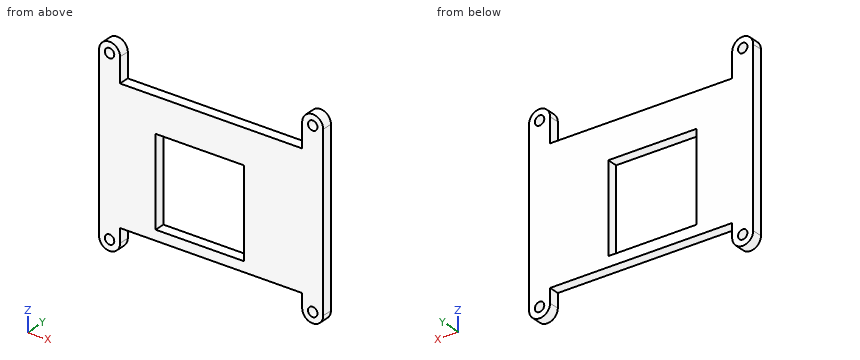
from build123d import *

# Parameters (mm, degrees)
SKETCH_1_R      = 1.35
SKETCH_1_W      = 25.2
SKETCH_1_H      = 25.2
EXTRUDE_1_DEPTH = 3


with BuildPart() as part:
    # 草图1 → 凸台-拉伸1 (new body)
    with BuildSketch(Plane(origin=(0, 0, 0), x_dir=(1, 0, 0), z_dir=(0, 1, 0))):
        with BuildLine():
            Line((-28.75, 19.5), (-28.75, -29.5))
            ThreePointArc((-28.75, -29.5), (-25.75, -32.5), (-22.75, -29.5))
            Line((-22.75, -29.5), (-22.75, -22.5))
            Line((-22.75, -22.5), (29.25, -22.5))
            Line((29.25, -22.5), (29.25, -29.5))
            ThreePointArc((29.25, -29.5), (32.25, -32.5), (35.25, -29.5))
            Line((35.25, -29.5), (35.25, 19.5))
            ThreePointArc((35.25, 19.5), (32.25, 22.5), (29.25, 19.5))
            Line((29.25, 19.5), (29.25, 15.5))
            Line((29.25, 15.5), (-22.75, 15.5))
            Line((-22.75, 15.5), (-22.75, 19.5))
            ThreePointArc((-22.75, 19.5), (-25.75, 22.5), (-28.75, 19.5))
        make_face()
        with Locations((-25.75, 19.5)):
            Circle(SKETCH_1_R, mode=Mode.SUBTRACT)
        with Locations((-25.75, -29.5)):
            Circle(SKETCH_1_R, mode=Mode.SUBTRACT)
        with Locations((32.25, 19.5)):
            Circle(SKETCH_1_R, mode=Mode.SUBTRACT)
        with Locations((32.25, -29.5)):
            Circle(SKETCH_1_R, mode=Mode.SUBTRACT)
        Rectangle(SKETCH_1_W, SKETCH_1_H, mode=Mode.SUBTRACT)
    extrude(amount=EXTRUDE_1_DEPTH)


solid = part.part
Could you check a few things on this model? Use its own coordinates, in mm. Give positions to 0.01 mm unless a question says otherwise; leave off trailing zeros. Write each loop counter-clockwise with the first axis right and the second up, starting at its lowest first coordinate (ties: lowest second). Pieces come first, ordered by that corner, then holes. Notation, with made-up numbers: (83, 28) -> (120, 28) arc R23 cw to (120, 55) -> close; hole circle Ø2 at (-39.5, 7.25). An arc over 180 degrees is marked (long way). Answer as CSV lines item,"result". Start each with the question number.
(1) If we section it at B-B, the plane x = 32.25: Write out the boundary of the cut face in (y, z), and give its area (3 significant figures).
(2) Please list where these lines run through material, in increasing order: line 1 (X direction, y = 1.45, z = 29.5); line 2 (Z direction, x = 32.25, y = 2.25).
(3) If we section it at A-A, the plane z = -3: Write out the boundary of the cut face in (x, y), and give its area (3 significant figures).
(4) If we section it at C-C, the plane y = 1.15: Write out the boundary of the cut face in (x, z).
(5) I'm going to push flat-ended pins straight in: pin 1 Ø1.5 at (x, y) = (-18.5, 1) entering from -Z; pin 2 Ø0.9 at (x, y) = (2, 2) entering from +Z. Where does each tip first touch, or does it pass through?
(6) If we section it at D-D, the plane x = 10: Write out the boundary of the cut face in (y, z), and give its area (3 significant figures).
Answer list:
1,outline,"(0, -22.5) -> (3, -22.5) -> (3, -20.85) -> (0, -20.85) -> close; (0, -18.15) -> (3, -18.15) -> (3, 28.15) -> (0, 28.15) -> close; (0, 30.85) -> (3, 30.85) -> (3, 32.5) -> (0, 32.5) -> close"
1,area,"149 mm^2"
2,line 1,"-28.75 to -27.1, -24.4 to -22.75, 29.25 to 30.9, 33.6 to 35.25"
2,line 2,"-22.5 to -20.85, -18.15 to 28.15, 30.85 to 32.5"
3,outline,"(-28.75, 0) -> (-12.6, 0) -> (-12.6, 3) -> (-28.75, 3) -> close; (12.6, 0) -> (35.25, 0) -> (35.25, 3) -> (12.6, 3) -> close"
3,area,"116 mm^2"
4,outline,"(-28.75, -19.5) arc R3 ccw to (-22.75, -19.5) -> (-22.75, -15.5) -> (29.25, -15.5) -> (29.25, -19.5) arc R3 ccw to (35.25, -19.5) -> (35.25, 29.5) arc R3 ccw to (29.25, 29.5) -> (29.25, 22.5) -> (-22.75, 22.5) -> (-22.75, 29.5) arc R3 ccw to (-28.75, 29.5) -> close; hole circle Ø2.7 at (-25.75, -19.5); hole circle Ø2.7 at (-25.75, 29.5); hole (-12.6, -12.6) -> (12.6, -12.6) -> (12.6, 12.6) -> (-12.6, 12.6) -> close; hole circle Ø2.7 at (32.25, -19.5); hole circle Ø2.7 at (32.25, 29.5)"
5,pin 1,"z = -15.5"
5,pin 2,"z = 22.5"
6,outline,"(0, -15.5) -> (3, -15.5) -> (3, -12.6) -> (0, -12.6) -> close; (0, 12.6) -> (3, 12.6) -> (3, 22.5) -> (0, 22.5) -> close"
6,area,"38.4 mm^2"
